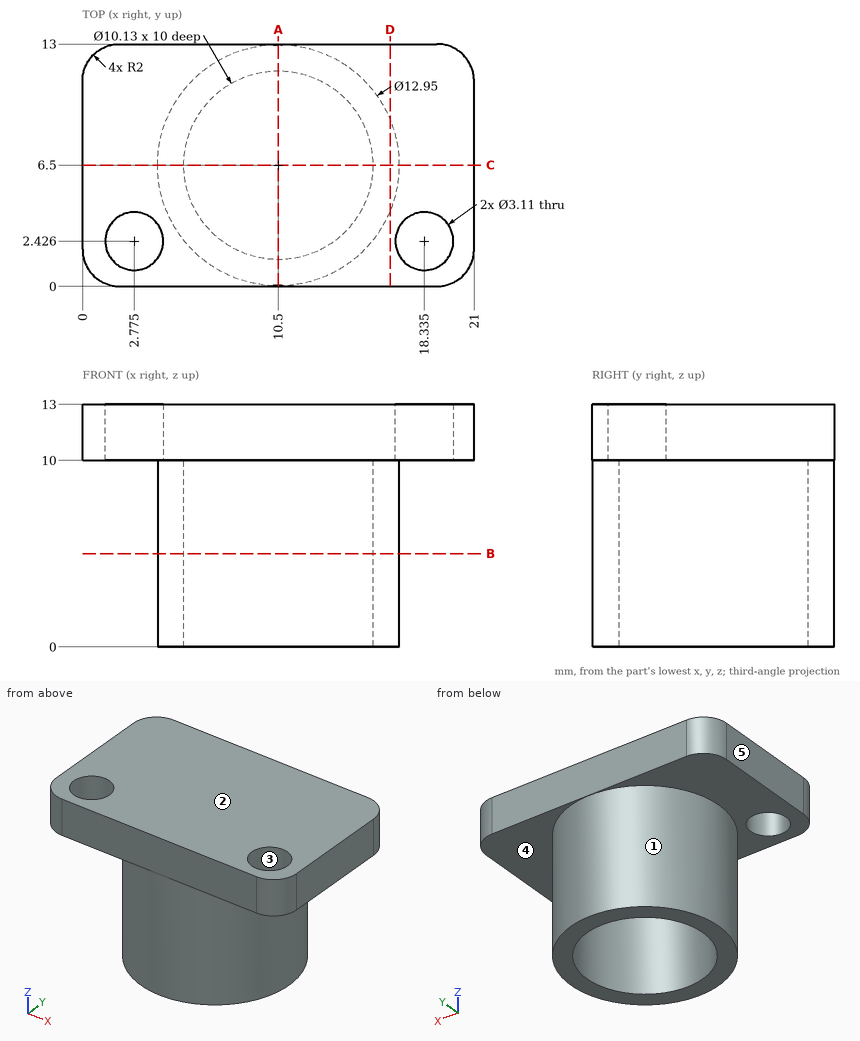
Part print with two shaded views. Sizes in mm from the minimum x, y, z corner. A direction names the side the tool comes from. Round coordinates to 2 decimals unless told otherwise and drop trailing zeros. Order: outer loops, then holes, each group sorted by start corner. A loop starts at its lowest first (then second) coordinate and runs counter-clockwise, first axis right, second up. Notation, with made-up numbers: (41, 2) - (62, 2) arc R14 ccw to (62, 23) - close; hole circle Ø10 at (86.5, 6). An arc over 180 degrees is marked (long way). Answer as CSV lines item,"result". Start each with the question number.
1. Saw through at B-B, the plane z = 5. Write the cut outline in (x, y) (3 decimals).
2. Pull direction X, two halves, no side cores. Call the marked faces 3, 4 and 5: +X half, -X half, draft (parallel to the pull), parting line (faces both ways), or undercut.
3. Tool access for the marked faces 1 and 2: list every direction of +Z, -Z, +X, -X, +Y, -Y with a clear straight run to the whole face (end or side of a thin tool).
4. Saw through at D-D, the plane x = 16.5. Write the cut outline in (y, z).
5. Pin check, flat tips, straight feed: pin 1 (1.5 mm diameter, centred on x = 2.5, y = 3, fed in from -Z); pin 2 (3 mm diameter, centred on x = 8.5, y = 7, fed in from -Z); pin 3 (3 mm diameter, centred on x = 14, z = 1.5, fed in from +Y); pin 4 (5 mm diameter, centred on x = 5.5, z = 7, fed in from -Y). Stop position of each tip, or through.
6. Saw through at A-A, the plane x = 10.5. Write the cut outline in (y, z) (3 decimals), and give its area (3 significant figures).
7. Drill centre lines: L1, parallel to Y at x = 10.5, z = 6.75 (3 decimals); L2, parallel to Z at x = 5.5, y = 12; L3, parallel to X at y = 10, z = 0.5. Where is each one in solid material? Low to high. Write a range as [from, to].
8. Saw through at C-C, the plane y = 6.5. Write the cut outline in (x, z) (3 decimals).
Model answer:
1,outline,"circle Ø12.95 at (10.5, 6.5); hole circle Ø10.13 at (10.5, 6.5)"
2,face 3,"undercut"
2,face 4,"draft"
2,face 5,"-X half"
3,face 1,"-Z"
3,face 2,"+Z, +X, -X, +Y, -Y"
4,outline,"(0, 10) - (4.07, 10) - (4.07, 0) - (8.93, 0) - (8.93, 10) - (13, 10) - (13, 13) - (0, 13) - close"
5,pin 1,"passes through"
5,pin 2,"stops at z = 10"
5,pin 3,"stops at y = 12.66"
5,pin 4,"stops at y = 0.53"
6,outline,"(0, 10) - (0.025, 10) - (0.025, 0) - (1.435, 0) - (1.435, 10) - (11.565, 10) - (11.565, 0) - (12.975, 0) - (12.975, 10) - (13, 10) - (13, 13) - (0, 13) - close"
6,area,"67.2 mm²"
7,L1,"y = [0.025, 1.435], [11.565, 12.975]"
7,L2,"z = [10, 13]"
7,L3,"x = [5.05, 6.84], [14.16, 15.95]"
8,outline,"(0, 10) - (4.025, 10) - (4.025, 0) - (5.435, 0) - (5.435, 10) - (15.565, 10) - (15.565, 0) - (16.975, 0) - (16.975, 10) - (21, 10) - (21, 13) - (0, 13) - close"
